Verification items for the finished model (mm, model axes). A direction names the side the tool comes from. Coordinates: 2 decimals unless noted, no trailing zeros. Write each loop counter-clockwise with the first axis right and the second up, starting at its lowest first coordinate (ties: lowest second). Pieces come first, ordered by that corner, then holes. Notation, with made-up numbers: (71.25, 12.25) - (130.25, 12.25) arc R25 cw to (130.25, 38.25) - close; hole circle Ø5 at (16, -2). An arc over 180 degrees is marked (long way). Use one line per item in the form item = value. Start each with the question number.
(1) Mould release check, pull along X, two halves, no side actions. Record for faces 4 (the flat face through (-60.236, 3, 0)), 5 (the cylindrical face through (35.117, 3.131, 34.477)), 6 (the cylindrical face through (41.22, 3.13, -0.18)): released by +X, released by -X, zero draft, split by the parting line, or undercut.
(2) Sectioned sample at B-B (x = 0). Record the cut outline in (y, z), and give its area (3 significant figures).
(3) Gauge pin test, flat ends, axial feed: pin 1 Ø13.5 at (x, z) = (-37.06, 0) entering from +Y; pin 2 Ø3 at (y, z) = (2.5, 56) entering from -X; pin 3 Ø2 at (y, z) = (1, 23.5) entering from -X; pin 4 Ø1.5 at (y, z) = (2.5, -24) entering from -X. Record the tip position at first contact, or that the pin passes through.
(4) Sectioned sample at C-C (y = 3.25). Count the separate pieces of the cut face and the enclosed holes in it, and give its area (3 significant figures).
(5) Material ranges on line 1 (Z direction, x = 0, y = 1.5); line 2 (X direction, y = 3.5, z = -3); line 3 (Z direction, x = 34, y = 4), recorded low to high. Write a range as [from, to].
(6) Tool access check on faces 1 (the flat face through (-55, 3, -6.35)), 2 (the flat face through (-55, 3, 6.35)), 3 (the flat face through (6.35, 3, -55)). Record the directions out of +Z, -Z, +X, -X, +Y, -Y that give a thin tool (end or side, any length) a straight path to the whole face; none if there is none.
(7) Sectioned sample at A-A (z = 0). Record the cut outline in (x, y).
(8) Sectioned sample at D-D (x = 38.5). Record the cut outline in (y, z), and give its area (3 significant figures).
Autodesk Inventor part; units mm, degrees
ref_plane "YZ Plane" through (0, 0, 0) normal (1, 0, 0) x (0, 1, 0)
ref_plane "XZ Plane" through (0, 0, 0) normal (0, 1, 0) x (-1, 0, 0)
ref_plane "XY Plane" through (0, 0, 0) normal (0, 0, 1) x (1, 0, 0)
sketch "Sketch1" plane through (0, 0, 0) normal (0, 1, 0) x (-1, 0, 0)
  circle A0 centre (53.5305, 0) radius 2.3813
  circle A1 centre (0, -53.5305) radius 2.3876
  circle A2 centre (-53.5305, 0) radius 2.3876
  circle A3 centre (0, 53.5305) radius 2.3876
  line L0 (0, 60.2361) -> (-6.35, 60.2361)
  line L1 (-6.35, 60.2361) -> (6.35, 60.2361)
  line L2 (6.35, 60.2361) -> (6.35, 48.8011)
  line L3 (-6.35, 60.2361) -> (-6.35, 48.8011)
  line L4 (-60.2361, 0) -> (-60.2361, -6.35)
  line L5 (-60.2361, -6.35) -> (-60.2361, 6.35)
  line L6 (-60.2361, 6.35) -> (-48.8011, 6.35)
  line L7 (-60.2361, -6.35) -> (-48.8011, -6.35)
  line L8 (0, -60.2361) -> (-6.35, -60.2361)
  line L9 (-6.35, -60.2361) -> (6.35, -60.2361)
  line L10 (6.35, -60.2361) -> (6.35, -48.8011)
  line L11 (-6.35, -60.2361) -> (-6.35, -48.8011)
  line L12 (60.2361, 0) -> (60.2361, -6.35)
  line L13 (60.2361, -6.35) -> (60.2361, 6.35)
  line L14 (60.2361, 6.35) -> (48.8011, 6.35)
  line L15 (60.2361, -6.35) -> (48.8011, -6.35)
  arc A4 (6.35, -48.8011) -> (48.8011, -6.35) centre (0, 0) ccw
  arc A5 (-48.8011, -6.35) -> (-6.35, -48.8011) centre (0, 0) ccw
  arc A6 (48.8011, 6.35) -> (6.35, 48.8011) centre (0, 0) ccw
  arc A7 (-6.35, 48.8011) -> (-48.8011, 6.35) centre (0, 0) ccw
  circle A8 centre (0, 0) radius 4.1656
  circle A9 centre (-37.0586, 0) radius 4.1656
  circle A10 centre (0, 37.0586) radius 4.1656
  circle A11 centre (37.0586, 0) radius 4.1656
  circle A12 centre (0, -37.0586) radius 4.1656
  dimension "d6" = 4.7625
  dimension "d7" = 4.7752
  dimension "d8" = 4.7752
  dimension "d9" = 4.7752
  dimension "d11" = 6.7056
  dimension "d12" = 6.7056
  dimension "d13" = 6.7056
  dimension "d14" = 6.7056
  dimension "d15" = 6.35
  dimension "d16" = 12.7
  dimension "d17" = 6.35
  dimension "d18" = 12.7
  dimension "d19" = 6.35
  dimension "d20" = 12.7
  dimension "d21" = 6.35
  dimension "d22" = 12.7
  dimension "d23" = 8.3312
  dimension "d29" = 8.3312
  dimension "d30" = 8.3312
  dimension "d31" = 8.3312
  dimension "d32" = 8.3312
extrude "Extrusion1" add sketch "Sketch1" along normal blind 6.35
properties part number "Rotating Base mount"
Answers below:
q1.face_4 = released by -X
q1.face_5 = released by +X
q1.face_6 = undercut
q2.outline = (0, -60.24) - (6.35, -60.24) - (6.35, -55.92) - (0, -55.92) - close; (0, -51.14) - (6.35, -51.14) - (6.35, -41.22) - (0, -41.22) - close; (0, -32.89) - (6.35, -32.89) - (6.35, -4.17) - (0, -4.17) - close; (0, 4.17) - (6.35, 4.17) - (6.35, 32.89) - (0, 32.89) - close; (0, 41.22) - (6.35, 41.22) - (6.35, 51.14) - (0, 51.14) - close; (0, 55.92) - (6.35, 55.92) - (6.35, 60.24) - (0, 60.24) - close
q2.area = 546 mm2
q3.pin_1 = 6.35
q3.pin_2 = -6.35
q3.pin_3 = -43.77
q3.pin_4 = -43.37
q4.separate_pieces = 1
q4.enclosed_holes = 9
q4.area = 7,830 mm2
q5.line_1 = [-60.24, -55.92], [-51.14, -41.22], [-32.89, -4.17], [4.17, 32.89], [41.22, 51.14], [55.92, 60.24]
q5.line_2 = [-60.24, -39.95], [-34.17, -2.89], [2.89, 34.17], [39.95, 60.24]
q5.line_3 = [-35.58, -2.83], [2.83, 35.58]
q6.face_1 = -Z, -X, +Y, -Y
q6.face_2 = +Z, -X, +Y, -Y
q6.face_3 = -Z, +X, +Y, -Y
q7.outline = (-60.24, 0) - (-55.91, 0) - (-55.91, 6.35) - (-60.24, 6.35) - close; (-51.15, 0) - (-41.22, 0) - (-41.22, 6.35) - (-51.15, 6.35) - close; (-32.89, 0) - (-4.17, 0) - (-4.17, 6.35) - (-32.89, 6.35) - close; (4.17, 0) - (32.89, 0) - (32.89, 6.35) - (4.17, 6.35) - close; (41.22, 0) - (51.14, 0) - (51.14, 6.35) - (41.22, 6.35) - close; (55.92, 0) - (60.24, 0) - (60.24, 6.35) - (55.92, 6.35) - close
q8.outline = (0, -30.65) - (6.35, -30.65) - (6.35, -3.91) - (0, -3.91) - close; (0, 3.91) - (6.35, 3.91) - (6.35, 30.65) - (0, 30.65) - close
q8.area = 340 mm2
